The model under review builds one solid part; all positions refer to its coordinate system, in mm. Face numbers are marked on the shaded views. A direction names the side the tool comes from. Coordinates: 2 decimals unless noted, no trailing zeros. Order: outer loops, then holes, each group sorted by start corner. A loop starts at its lowest first (then second) coordinate and runs counter-clockwise, first axis right, second up. Notation, with made-up numbers: (-25.75, 76) - (29.25, 76) arc R18 cw to (29.25, 88) - close; hole circle Ø9 at (10, 82). An arc over 180 degrees is marked (long way). Answer in a Markdown table with one row per item.
```python
from build123d import *

# Parameters (mm, degrees)
F1_DEPTH  = 10
F2_R      = 1.6
F3_DEPTH  = 40
F4_R      = 1.4
F5_DEPTH  = 40
F6_W      = 5
F6_H      = 10
F7_DEPTH  = 4
F8_R      = 0.8
F9_DEPTH  = 7
F10_R     = 0.9
F11_DEPTH = 1


with BuildPart() as f1:
    # F0 (on Front) → F1 (new body)
    with BuildSketch(Plane.XZ):
        with BuildLine():
            ThreePointArc((13.6747943312, 3), (13.9184611333, 1.5087874873), (14, 0))
            ThreePointArc((14, 0), (13.9184611333, -1.5087874873), (13.6747943312, -3))
            Line((13.6747943312, -3), (17.2409396496, -3))
            ThreePointArc((17.2409396496, -3), (17.4351146235, -1.5055823014), (17.5, 0))
            ThreePointArc((17.5, 0), (17.4351146235, 1.5055823014), (17.2409396496, 3))
            Line((17.2409396496, 3), (13.6747943312, 3))
        make_face()
        with BuildLine():
            ThreePointArc((3, 13.6747943312), (9.8994949366, 9.8994949366), (13.6747943312, 3))
            Line((13.6747943312, 3), (17.2409396496, 3))
            ThreePointArc((17.2409396496, 3), (12.3743686708, 12.3743686708), (3, 17.2409396496))
            Line((3, 17.2409396496), (3, 13.6747943312))
        make_face()
        with BuildLine():
            Line((17.2409396496, -3), (13.6747943312, -3))
            ThreePointArc((13.6747943312, -3), (9.8994949366, -9.8994949366), (3, -13.6747943312))
            Line((3, -13.6747943312), (3, -17.2409396496))
            ThreePointArc((3, -17.2409396496), (12.3743686708, -12.3743686708), (17.2409396496, -3))
        make_face()
        with BuildLine():
            ThreePointArc((-3, 13.6747943312), (0, 14), (3, 13.6747943312))
            Line((3, 13.6747943312), (3, 17.2409396496))
            ThreePointArc((3, 17.2409396496), (0, 17.5), (-3, 17.2409396496))
            Line((-3, 17.2409396496), (-3, 13.6747943312))
        make_face()
        with BuildLine():
            Line((18.5, 3), (17.2409396496, 3))
            ThreePointArc((17.2409396496, 3), (17.4351146235, 1.5055823014), (17.5, 0))
            ThreePointArc((17.5, 0), (17.4351146235, -1.5055823014), (17.2409396496, -3))
            Line((17.2409396496, -3), (18.5, -3))
            Line((18.5, -3), (18.5, 3))
        make_face()
        with BuildLine():
            Line((3, -17.2409396496), (3, -13.6747943312))
            ThreePointArc((3, -13.6747943312), (0, -14), (-3, -13.6747943312))
            Line((-3, -13.6747943312), (-3, -17.2409396496))
            ThreePointArc((-3, -17.2409396496), (0, -17.5), (3, -17.2409396496))
        make_face()
        with BuildLine():
            ThreePointArc((-13.6747943312, 3), (-9.8994949366, 9.8994949366), (-3, 13.6747943312))
            Line((-3, 13.6747943312), (-3, 17.2409396496))
            ThreePointArc((-3, 17.2409396496), (-12.3743686708, 12.3743686708), (-17.2409396496, 3))
            Line((-17.2409396496, 3), (-13.6747943312, 3))
        make_face()
        with BuildLine():
            ThreePointArc((-3, 17.2409396496), (0, 17.5), (3, 17.2409396496))
            Line((3, 17.2409396496), (3, 18.5))
            Line((3, 18.5), (-3, 18.5))
            Line((-3, 18.5), (-3, 17.2409396496))
        make_face()
        with BuildLine():
            Line((-3, -17.2409396496), (-3, -13.6747943312))
            ThreePointArc((-3, -13.6747943312), (-9.8994949366, -9.8994949366), (-13.6747943312, -3))
            Line((-13.6747943312, -3), (-17.2409396496, -3))
            ThreePointArc((-17.2409396496, -3), (-12.3743686708, -12.3743686708), (-3, -17.2409396496))
        make_face()
        with BuildLine():
            Line((3, -18.5), (3, -17.2409396496))
            ThreePointArc((3, -17.2409396496), (0, -17.5), (-3, -17.2409396496))
            Line((-3, -17.2409396496), (-3, -18.5))
            Line((-3, -18.5), (3, -18.5))
        make_face()
        with BuildLine():
            ThreePointArc((-13.6747943312, -3), (-14, 0), (-13.6747943312, 3))
            Line((-13.6747943312, 3), (-17.2409396496, 3))
            ThreePointArc((-17.2409396496, 3), (-17.5, 0), (-17.2409396496, -3))
            Line((-17.2409396496, -3), (-13.6747943312, -3))
        make_face()
        with BuildLine():
            ThreePointArc((-17.2409396496, -3), (-17.5, 0), (-17.2409396496, 3))
            Line((-17.2409396496, 3), (-18.5, 3))
            Line((-18.5, 3), (-18.5, -3))
            Line((-18.5, -3), (-17.2409396496, -3))
        make_face()
    extrude(amount=F1_DEPTH)

    # F2 (on face) → F3 (cut)
    with BuildSketch(Plane.XY.offset(18.5)):
        with Locations((0, -5)):
            Circle(F2_R)
    extrude(amount=-F3_DEPTH, mode=Mode.SUBTRACT)

    # F4 (on face) → F5 (cut)
    with BuildSketch(Plane.YZ.offset(18.5)):
        with Locations((-5, 0)):
            Circle(F4_R)
    extrude(amount=-F5_DEPTH, mode=Mode.SUBTRACT)

    # F6 (on face) → F7 (join)
    with BuildSketch(Plane.XY.offset(18.5)):
        with Locations((5.5, -5)):
            Rectangle(F6_W, F6_H)
    extrude(amount=-F7_DEPTH)

    # F8 (on face) → F9 (cut)
    with BuildSketch(Plane.XY.offset(18.5)):
        with Locations((5.5, -5)):
            Circle(F8_R)
    extrude(amount=-F9_DEPTH, mode=Mode.SUBTRACT)

    # F10 (on face) → F11 (cut)
    with BuildSketch(Plane.XY.offset(18.5)):
        with Locations((5.5, -5)):
            Circle(F10_R)
    extrude(amount=-F11_DEPTH, mode=Mode.SUBTRACT)


solid = f1.part
```
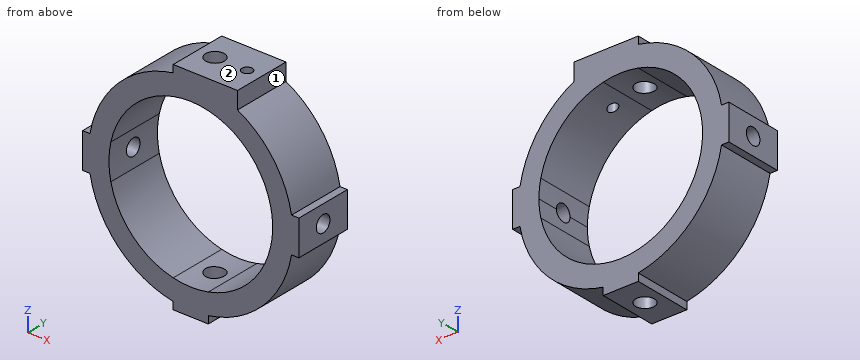
Item 1: Clearance check with flat-ended pins moving along their axes: pin 1 Ø0.9 at (y, z) = (-4.5, 16.5) entering from +X; pin 2 Ø3 at (y, z) = (-5, 0) entering from +X; pin 3 Ø1.1 at (x, y) = (5.5, -5) entering from +Z; pin 4 Ø0.6 at (y, z) = (-4, -18) entering from -X. State where each tip first meets the part, or that it passes through.
Check values:
| item | result |
|---|---|
| pin 1 | x = 8 |
| pin 2 | x = 18.5 |
| pin 3 | z = -12.63 |
| pin 4 | x = -3 |
Item 2: We need section C-C, the plane y = -8.25. Write out the cut boundary in (x, z), then the cut area to 3 significant figures.
Check values:
| item | result |
|---|---|
| outline | (-18.5, -3) - (-17.24, -3) arc R17.5 ccw to (-3, -17.24) - (-3, -18.5) - (3, -18.5) - (3, -17.24) arc R17.5 ccw to (17.24, -3) - (18.5, -3) - (18.5, 3) - (17.24, 3) arc R17.5 ccw to (8, 15.56) - (8, 18.5) - (-3, 18.5) - (-3, 17.24) arc R17.5 ccw to (-17.24, 3) - (-18.5, 3) - close; hole circle Ø28 at (0, 0) |
| area | 382 mm^2 |
Item 3: We need section B-B, the plane x = 4. Write out the cut boundary in (y, z), then the cut area to 3 significant figures.
Check values:
| item | result |
|---|---|
| outline | (-10, -17.04) - (0, -17.04) - (0, -13.42) - (-10, -13.42) - close; (-10, 13.42) - (0, 13.42) - (0, 18.5) - (-10, 18.5) - close |
| area | 87.0 mm^2 |
Item 4: To check wall thickness, follow line 1 (X direction, y = -5, z = 15.85); line 2 (X direction, y = -8.75, z = 0); line 3 (Y direction, x = 16, z = 0). State the ranges of each line that lie inside material, in increasing order. Write a range as from..to.
Check values:
| item | result |
|---|---|
| line 1 | -7.42..-1.6, 1.6..4.7, 6.3..8 |
| line 2 | -18.5..-14, 14..18.5 |
| line 3 | -10..-6.4, -3.6..0 |
Item 5: We need section A-A, the plane x = 0. Write out the cut boundary in (y, z).
Check values:
| item | result |
|---|---|
| outline | (-10, -18.5) - (-6.6, -18.5) - (-6.6, -14) - (-10, -14) - close; (-10, 14) - (-6.6, 14) - (-6.6, 18.5) - (-10, 18.5) - close; (-3.4, -18.5) - (0, -18.5) - (0, -14) - (-3.4, -14) - close; (-3.4, 14) - (0, 14) - (0, 18.5) - (-3.4, 18.5) - close |
Item 6: We need section D-D, the plane z = -6.5. Write out the cut boundary in (x, y), then the cut area to 3 significant figures.
Check values:
| item | result |
|---|---|
| outline | (-16.25, -10) - (-12.4, -10) - (-12.4, 0) - (-16.25, 0) - close; (12.4, -10) - (16.25, -10) - (16.25, 0) - (12.4, 0) - close |
| area | 77.0 mm^2 |
Item 7: Tool access review of the marked faces 1 and 2: name each direction out of +Z, -Z, +X, -X, +Y, -Y from which nothing blocks a thin tool from reaching the whole face with its end or side.
Check values:
| item | result |
|---|---|
| face 1 | +Z, +X, +Y, -Y |
| face 2 | +Z, +X, -X, +Y, -Y |
